Could you check a few things on this model? Use its own coordinates, in mm. Give positions to 0.01 mm unless a question says otherwise; leave off trailing zeros. Order: outer loops, then holes, each group sorted by start corner. A loop starts at its lowest first (then second) coordinate and runs counter-clockwise, first axis right, second up.
(1) If I drill on probe 1 along X at (y, z) = (1.7, -93.5); probe 2 along Z at (x, y) = (2.5, 0.9); probe 3 along X at (y, z) = (0.75, -80), over which ranges is the centre line in solid material (lowest first)?
(2) Imagine slicing it at A-A, the plane z = -80. Write out the boundary of the cut face in (x, y) (3 decimals), then the cut area to 3 significant figures.
(3) Imagine slicing it at C-C, the plane z = -93.5. Write out the boundary of the cut face in (x, y) (3 decimals).
(4) Will this pin go through, and if not, where does the flat tip stop? pin 1 (2 mm diameter, centred on x = 13, z = -47, fed in from -Y).
(5) Imagine slicing it at B-B, the plane x = 16.5. Write out the boundary of the cut face in (y, z) (3 decimals).
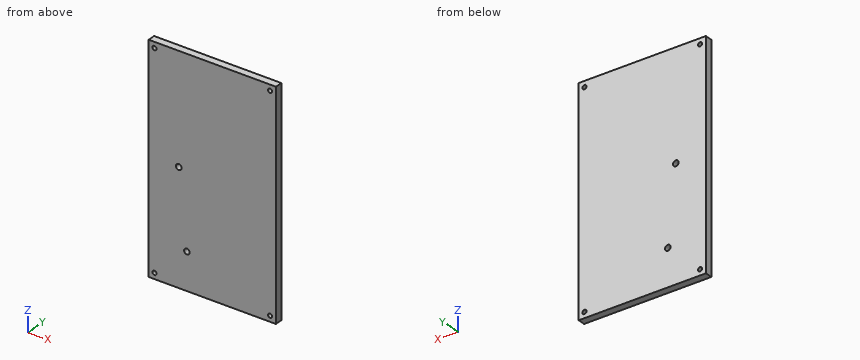
from build123d import *

# Parameters (mm, degrees)
SKETCH2_W             = 55
SKETCH2_H             = 96
BOSS_EXTRUDE1_DEPTH   = 3.175
F_2_CLEARANCE_HOLE1_D = 2.4384
F_0_CLEARANCE_HOLE1_D = 1.778


with BuildPart() as part:
    # Sketch2 → Boss-Extrude1 (new body)
    with BuildSketch(Plane(origin=(0, 0, 0), x_dir=(1, 0, 0), z_dir=(0, 1, 0))):
        with Locations((27.5, 48)):
            Rectangle(SKETCH2_W, SKETCH2_H)
    extrude(amount=BOSS_EXTRUDE1_DEPTH)

    # #2 Clearance Hole1 (through all)
    with Locations(Plane(origin=(0, 3.175, 0), x_dir=(1, 0, 0), z_dir=(0, 1, 0))):
        with Locations((16.5, 80), (13, 47)):
            Hole(F_2_CLEARANCE_HOLE1_D / 2)

    # #0 Clearance Hole1 (through all)
    with Locations(Plane(origin=(0, 3.175, 0), x_dir=(1, 0, 0), z_dir=(0, 1, 0))):
        with Locations((2.5, 2.5), (52.5, 2.5), (52.5, 93.5), (2.5, 93.5)):
            Hole(F_0_CLEARANCE_HOLE1_D / 2)


solid = part.part
Answer block:
1. probe 1: x = 0 to 1.61, 3.39 to 51.61, 53.39 to 55
1. probe 2: z = -96 to -94.39, -92.61 to -3.39, -1.61 to 0
1. probe 3: x = 0 to 15.28, 17.72 to 55
2. outline: (0, 0) - (15.281, 0) - (15.281, 3.175) - (0, 3.175) - close; (17.719, 0) - (55, 0) - (55, 3.175) - (17.719, 3.175) - close
2. area: 167 mm2
3. outline: (0, 0) - (1.611, 0) - (1.611, 3.175) - (0, 3.175) - close; (3.389, 0) - (51.611, 0) - (51.611, 3.175) - (3.389, 3.175) - close; (53.389, 0) - (55, 0) - (55, 3.175) - (53.389, 3.175) - close
4. pin 1: passes through
5. outline: (0, -96) - (3.175, -96) - (3.175, -81.219) - (0, -81.219) - close; (0, -78.781) - (3.175, -78.781) - (3.175, 0) - (0, 0) - close
